Read the model definition and answer for the solid it produces. Units are mm, in the model's axes. Coordinates: 2 decimals unless noted, no trailing zeros. Order: outer loops, then holes, each group sorted by start corner. A loop starts at its lowest first (then second) coordinate and runs counter-clockwise, first axis right, second up. Notation, with made-up numbers: (76, -2) -> (99, -2) arc R20 cw to (99, 7) -> close; hole circle Ø1 at (12, 25). An arc over 180 degrees is marked (long way). Use CSV: the item, a comma, the result in double quotes.
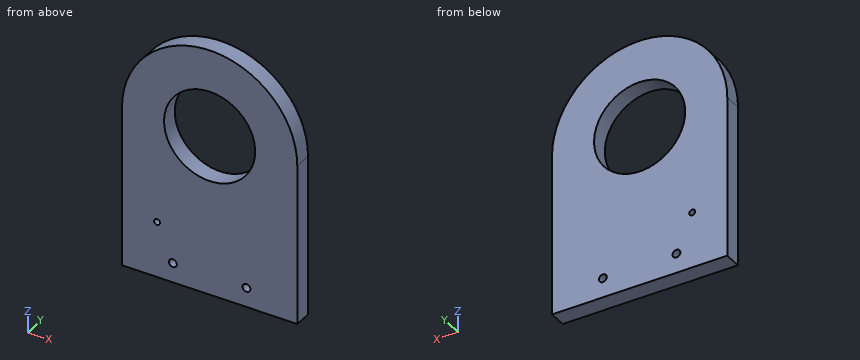
```python
from build123d import *

# Parameters (mm, degrees)
PARED_START               = 29.75
SK_PARED_W                = 100
SK_PARED_H                = 92
PARED_DEPTH               = 10
CABEZA_START              = 29.75
SK_CABEZA_R               = 50
CABEZA_DEPTH              = 10
PASO_CUBO_J2_START        = 29.75
SK_PASO_CUBO_J2_R         = 26
PASO_CUBO_J2_DEPTH        = 10
PASANTES_M4_ANGULOS_START = 29.75
SK_PASANTES_M4_ANGULOS_R  = 2.25
PASANTES_M4_ANGULOS_DEPTH = 10
PASANTE_M3_CINCHO_START   = 29.75
SK_PASANTE_M3_CINCHO_R    = 1.7
PASANTE_M3_CINCHO_DEPTH   = 10


with BuildPart() as part:
    # Sk_Pared → Pared (new body)
    with BuildSketch(Plane(origin=(0, 0, 0), x_dir=(1, 0, 0), z_dir=(0, 1, 0)).offset(PARED_START)):
        with Locations((0, -124)):
            Rectangle(SK_PARED_W, SK_PARED_H)
    extrude(amount=PARED_DEPTH)

    # Sk_Cabeza → Cabeza (add)
    with BuildSketch(Plane(origin=(0, 0, 0), x_dir=(1, 0, 0), z_dir=(0, 1, 0)).offset(CABEZA_START)):
        with Locations((0, -170)):
            Circle(SK_CABEZA_R)
    extrude(amount=CABEZA_DEPTH)

    # Sk_Paso_cubo_J2 → Paso_cubo_J2 (cut)
    with BuildSketch(Plane(origin=(0, 0, 0), x_dir=(1, 0, 0), z_dir=(0, 1, 0)).offset(PASO_CUBO_J2_START)):
        with Locations(Location((0, -170, 0), (0, 0, 270))):
            Circle(SK_PASO_CUBO_J2_R)
    extrude(amount=PASO_CUBO_J2_DEPTH, mode=Mode.SUBTRACT)

    # Sk_Pasantes_M4_angulos → Pasantes_M4_angulos (cut)
    with BuildSketch(Plane(origin=(0, 0, 0), x_dir=(1, 0, 0), z_dir=(0, 1, 0)).offset(PASANTES_M4_ANGULOS_START)):
        with Locations(Location((-21, -89.11, 0), (0, 0, 270))):
            Circle(SK_PASANTES_M4_ANGULOS_R)
        with Locations(Location((21, -89.11, 0), (0, 0, 270))):
            Circle(SK_PASANTES_M4_ANGULOS_R)
    extrude(amount=PASANTES_M4_ANGULOS_DEPTH, mode=Mode.SUBTRACT)

    # Sk_Pasante_M3_cincho → Pasante_M3_cincho (cut)
    with BuildSketch(Plane(origin=(0, 0, 0), x_dir=(1, 0, 0), z_dir=(0, 1, 0)).offset(PASANTE_M3_CINCHO_START)):
        with Locations(Location((-30, -110, 0), (0, 0, 270))):
            Circle(SK_PASANTE_M3_CINCHO_R)
    extrude(amount=PASANTE_M3_CINCHO_DEPTH, mode=Mode.SUBTRACT)


solid = part.part
```
Item 1: Find section A-A, the plane x = -30. Give the vertices of the cut face in (y, z).
Return value:
outline,"(29.75, 78) -> (39.75, 78) -> (39.75, 108.3) -> (29.75, 108.3) -> close; (29.75, 111.7) -> (39.75, 111.7) -> (39.75, 210) -> (29.75, 210) -> close"
Item 2: Find section D-D, the plane z = 89.11. Give the vertices of the cut face in (x, y), then the cut area to 3 significant figures.
Return value:
outline,"(-50, 29.75) -> (-23.25, 29.75) -> (-23.25, 39.75) -> (-50, 39.75) -> close; (-18.75, 29.75) -> (18.75, 29.75) -> (18.75, 39.75) -> (-18.75, 39.75) -> close; (23.25, 29.75) -> (50, 29.75) -> (50, 39.75) -> (23.25, 39.75) -> close"
area,"910 mm^2"
Item 3: Straight lines are drawn through the part: line 1 along X through (y, z) = (37.5, 89.11); line 2 along X through (y, z) = (32, 170); line 3 along Z through (x, y) = (22.5, 38.5). For each, find the intervals that lie inside material, in ascending order.
Return value:
line 1,"x = -50 to -23.25, -18.75 to 18.75, 23.25 to 50"
line 2,"x = -50 to -26, 26 to 50"
line 3,"z = 78 to 87.43, 90.79 to 156.97, 183.03 to 214.65"
Item 4: Find section C-C, the plane y = 35.25. Give the vertices of the cut face in (x, z).
Return value:
outline,"(-50, 78) -> (50, 78) -> (50, 170) arc R50 ccw to (-50, 170) -> close; hole circle Ø3.4 at (-30, 110); hole circle Ø52 at (0, 170); hole circle Ø4.5 at (-21, 89.11); hole circle Ø4.5 at (21, 89.11)"
Item 5: Find section B-B, the plane z = 110. Give the vertices of the cut face in (x, y), then the cut area to 3 significant figures.
Return value:
outline,"(-50, 29.75) -> (-31.7, 29.75) -> (-31.7, 39.75) -> (-50, 39.75) -> close; (-28.3, 29.75) -> (50, 29.75) -> (50, 39.75) -> (-28.3, 39.75) -> close"
area,"966 mm^2"
Item 6: This flat-tipped pin is pushed along its axis until it touches: P1, Ø2, axis at x = -28.5, y = 37.5, coming from the +Z side. Where does it stop, or does it pass through?
Return value:
P1,"stops at z = 211.76"
